from build123d import *

# Parameters (mm, degrees)
SKETCH1_R           = 17
BOSS_EXTRUDE1_DEPTH = 15
CUT_EXTRUDE2_DEPTH  = 5
SKETCH3_R           = 1.75
CUT_EXTRUDE3_DEPTH  = 5
SKETCH4_W           = 3
SKETCH4_H           = 4
SKETCH5_R           = 6.36
CUT_EXTRUDE4_DEPTH  = 3.3


with BuildPart() as part:
    # Sketch1 → Boss-Extrude1 (new body)
    with BuildSketch(Plane.XY):
        Circle(SKETCH1_R)
    extrude(amount=BOSS_EXTRUDE1_DEPTH)

    # Sketch2 → Cut-Extrude2 (cut)
    with BuildSketch(Plane(origin=(0, 0, 0), x_dir=(-1, 0, 0), z_dir=(0, 0, -1))):
        with BuildLine():
            ThreePointArc((5.676819497, 7.303165094), (3.539821749, 8.545885676), (1.15, 9.178235124))
            ThreePointArc((1.15, 9.178235124), (0, 8.028235124), (-1.15, 9.178235124))
            ThreePointArc((-1.15, 9.178235124), (-3.539821749, 8.545885676), (-5.676819497, 7.303165094))
            ThreePointArc((-5.676819497, 7.303165094), (-5.676819497, 5.676819497), (-7.303165094, 5.676819497))
            ThreePointArc((-7.303165094, 5.676819497), (-8.545885676, 3.539821749), (-9.178235124, 1.15))
            ThreePointArc((-9.178235124, 1.15), (-8.028235124, 0), (-9.178235124, -1.15))
            ThreePointArc((-9.178235124, -1.15), (-8.545885676, -3.539821749), (-7.303165094, -5.676819497))
            ThreePointArc((-7.303165094, -5.676819497), (-5.676819497, -5.676819497), (-5.676819497, -7.303165094))
            ThreePointArc((-5.676819497, -7.303165094), (-3.539821749, -8.545885676), (-1.15, -9.178235124))
            ThreePointArc((-1.15, -9.178235124), (0, -8.028235124), (1.15, -9.178235124))
            ThreePointArc((1.15, -9.178235124), (3.539821749, -8.545885676), (5.676819497, -7.303165094))
            ThreePointArc((5.676819497, -7.303165094), (5.676819497, -5.676819497), (7.303165094, -5.676819497))
            ThreePointArc((7.303165094, -5.676819497), (8.545885676, -3.539821749), (9.178235124, -1.15))
            ThreePointArc((9.178235124, -1.15), (8.028235124, 0), (9.178235124, 1.15))
            ThreePointArc((9.178235124, 1.15), (8.545885676, 3.539821749), (7.303165094, 5.676819497))
            ThreePointArc((7.303165094, 5.676819497), (5.676819497, 5.676819497), (5.676819497, 7.303165094))
        make_face()
        with BuildLine():
            Line((9.333809512, 10.960155108), (5.676819497, 7.303165094))
            ThreePointArc((5.676819497, 7.303165094), (6.540737726, 6.540737726), (7.303165094, 5.676819497))
            Line((7.303165094, 5.676819497), (10.960155108, 9.333809512))
            ThreePointArc((10.960155108, 9.333809512), (10.960155108, 10.960155108), (9.333809512, 10.960155108))
        make_face()
        with BuildLine():
            Line((14.35, 1.15), (9.178235124, 1.15))
            ThreePointArc((9.178235124, 1.15), (9.232041348, 0.57611852), (9.25, 0))
            ThreePointArc((9.25, 0), (9.232041348, -0.57611852), (9.178235124, -1.15))
            Line((9.178235124, -1.15), (14.35, -1.15))
            ThreePointArc((14.35, -1.15), (15.5, 0), (14.35, 1.15))
        make_face()
        with BuildLine():
            Line((10.960155108, -9.333809512), (7.303165094, -5.676819497))
            ThreePointArc((7.303165094, -5.676819497), (6.540737726, -6.540737726), (5.676819497, -7.303165094))
            Line((5.676819497, -7.303165094), (9.333809512, -10.960155108))
            ThreePointArc((9.333809512, -10.960155108), (10.960155108, -10.960155108), (10.960155108, -9.333809512))
        make_face()
        with BuildLine():
            Line((1.15, -14.35), (1.15, -9.178235124))
            ThreePointArc((1.15, -9.178235124), (0, -9.25), (-1.15, -9.178235124))
            Line((-1.15, -9.178235124), (-1.15, -14.35))
            ThreePointArc((-1.15, -14.35), (0, -15.5), (1.15, -14.35))
        make_face()
        with BuildLine():
            ThreePointArc((-5.676819497, -7.303165094), (-6.540737726, -6.540737726), (-7.303165094, -5.676819497))
            Line((-7.303165094, -5.676819497), (-10.960155108, -9.333809512))
            ThreePointArc((-10.960155108, -9.333809512), (-10.960155108, -10.960155108), (-9.333809512, -10.960155108))
            Line((-9.333809512, -10.960155108), (-5.676819497, -7.303165094))
        make_face()
        with BuildLine():
            ThreePointArc((-9.178235124, -1.15), (-9.25, 0), (-9.178235124, 1.15))
            Line((-9.178235124, 1.15), (-14.35, 1.15))
            ThreePointArc((-14.35, 1.15), (-15.5, 0), (-14.35, -1.15))
            Line((-14.35, -1.15), (-9.178235124, -1.15))
        make_face()
        with BuildLine():
            ThreePointArc((-7.303165094, 5.676819497), (-6.540737726, 6.540737726), (-5.676819497, 7.303165094))
            Line((-5.676819497, 7.303165094), (-9.333809512, 10.960155108))
            ThreePointArc((-9.333809512, 10.960155108), (-10.960155108, 10.960155108), (-10.960155108, 9.333809512))
            Line((-10.960155108, 9.333809512), (-7.303165094, 5.676819497))
        make_face()
        with BuildLine():
            Line((1.15, 9.178235124), (1.15, 14.35))
            ThreePointArc((1.15, 14.35), (0, 15.5), (-1.15, 14.35))
            Line((-1.15, 14.35), (-1.15, 9.178235124))
            ThreePointArc((-1.15, 9.178235124), (0, 9.25), (1.15, 9.178235124))
        make_face()
        with BuildLine():
            ThreePointArc((5.676819497, -7.303165094), (6.540737726, -6.540737726), (7.303165094, -5.676819497))
            ThreePointArc((7.303165094, -5.676819497), (5.676819497, -5.676819497), (5.676819497, -7.303165094))
        make_face()
        with BuildLine():
            ThreePointArc((-1.15, 9.178235124), (0, 8.028235124), (1.15, 9.178235124))
            ThreePointArc((1.15, 9.178235124), (0, 9.25), (-1.15, 9.178235124))
        make_face()
        with BuildLine():
            ThreePointArc((7.303165094, 5.676819497), (6.540737726, 6.540737726), (5.676819497, 7.303165094))
            ThreePointArc((5.676819497, 7.303165094), (5.676819497, 5.676819497), (7.303165094, 5.676819497))
        make_face()
        with BuildLine():
            ThreePointArc((9.25, 0), (9.232041348, 0.57611852), (9.178235124, 1.15))
            ThreePointArc((9.178235124, 1.15), (8.028235124, 0), (9.178235124, -1.15))
            ThreePointArc((9.178235124, -1.15), (9.232041348, -0.57611852), (9.25, 0))
        make_face()
        with BuildLine():
            ThreePointArc((-1.15, -9.178235124), (0, -9.25), (1.15, -9.178235124))
            ThreePointArc((1.15, -9.178235124), (0, -8.028235124), (-1.15, -9.178235124))
        make_face()
        with BuildLine():
            ThreePointArc((-5.676819497, -7.303165094), (-5.676819497, -5.676819497), (-7.303165094, -5.676819497))
            ThreePointArc((-7.303165094, -5.676819497), (-6.540737726, -6.540737726), (-5.676819497, -7.303165094))
        make_face()
        with BuildLine():
            ThreePointArc((-9.178235124, -1.15), (-8.028235124, 0), (-9.178235124, 1.15))
            ThreePointArc((-9.178235124, 1.15), (-9.25, 0), (-9.178235124, -1.15))
        make_face()
        with BuildLine():
            ThreePointArc((-7.303165094, 5.676819497), (-5.676819497, 5.676819497), (-5.676819497, 7.303165094))
            ThreePointArc((-5.676819497, 7.303165094), (-6.540737726, 6.540737726), (-7.303165094, 5.676819497))
        make_face()
    extrude(amount=-CUT_EXTRUDE2_DEPTH, mode=Mode.SUBTRACT)

    # Sketch3 → Cut-Extrude3 (cut)
    with BuildSketch(Plane.XY.offset(15)):
        with Locations((0, 9.78)):
            Circle(SKETCH3_R)
        with Locations((9.78, 0)):
            Circle(SKETCH3_R)
        with Locations((0, -9.78)):
            Circle(SKETCH3_R)
        with Locations((-9.78, 0)):
            Circle(SKETCH3_R)
    extrude(amount=-CUT_EXTRUDE3_DEPTH, mode=Mode.SUBTRACT)

    # Sketch4 → Revolve1 (revolve)
    with BuildSketch(Plane(origin=(0, 0, 0), x_dir=(0, 0, -1), z_dir=(1, 0, 0))):
        with Locations((-7.5, -19)):
            Rectangle(SKETCH4_W, SKETCH4_H)
    revolve(axis=Axis((0, 0, 20.375620023), (0, 0, -1)))

    # Sketch5 → Cut-Extrude4 (cut)
    with BuildSketch(Plane.XY.offset(15)):
        Circle(SKETCH5_R)
    extrude(amount=-CUT_EXTRUDE4_DEPTH, mode=Mode.SUBTRACT)


solid = part.part
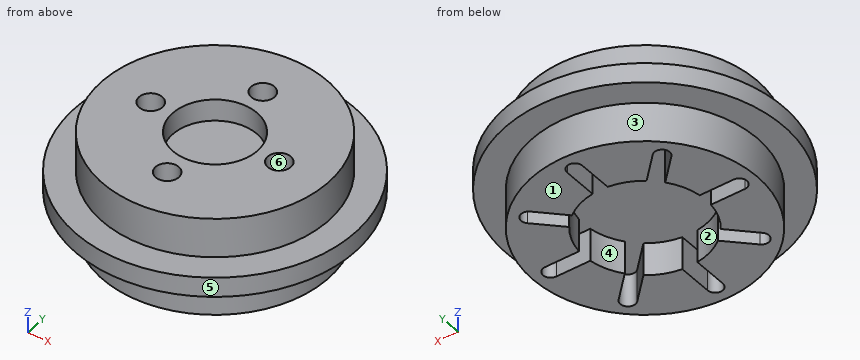
The model under review builds one solid part; all positions refer to its coordinate system, in mm. Face numbers are marked on the shaded views. A direction names the side the tool comes from. Coordinates: 2 decimals unless noted, no trailing zeros. Loops run counter-clockwise (first coordinate to the right, second up) from the corner with the lowest first, then second, coordinate; pieces in that order, holes last. Notation, with made-up numbers: (-29.75, 52) -> (23.25, 52) arc R16 cw to (23.25, 57) -> close; hole circle Ø9 at (-26.75, 9). An arc over 180 degrees is marked (long way). Use a Markdown table: item, result. Add a question column.
1. Add section D-D on y = 4. Write out the cut boundary in (x, z).
2. Add section C-C on z = 12.5. Write out the cut boundary in (x, y).
3. To check wall thickness, follow line 1 (Y direction, x = 0, z = 11.75); line 2 (X direction, y = -11, z = 4); line 3 (Y direction, x = 8, z = 1.5). State the ranges of each line that lie inside material, in increasing order.
4. Clearance check with flat-ended pins moving along their axes: pin 1 Ø1 at (x, z) = (-15.5, 12) entering from -Y; pin 2 Ø10 at (x, y) = (0, 0) entering from -Z; pin 3 Ø3 at (x, y) = (-9.78, 0) entering from +Z. State where each tip first meets the part, or that it passes through.
5. Machinability: for the marked faces 4, 5 and 6, which of the approach directions +Z, -Z, +X, -X, +Y, -Y give a long, thin tool a straight path to every point of the face, cutting with its end or side? Answer none if there is none.
6. Add section A-A on x = 0. Write out the cut boundary in (y, z), plus the area to 3 significant figures.
7. Draft analysis for pull direction X (two halves, no side actions). For the marked faces 1, 2 and 3, state which applies: pulls with the +X half, pulls with the -X half, needs draft (parallel to the pull), parting line crosses it, or undercut.
Returned:
| question | item | result |
|---|---|---|
| 1 | outline | (-20.62, 6) -> (-16.52, 6) -> (-16.52, 0) -> (-8.34, 0) -> (-8.34, 5) -> (8.34, 5) -> (8.34, 0) -> (16.52, 0) -> (16.52, 6) -> (20.62, 6) -> (20.62, 9) -> (16.52, 9) -> (16.52, 15) -> (4.94, 15) -> (4.94, 11.7) -> (-4.94, 11.7) -> (-4.94, 15) -> (-16.52, 15) -> (-16.52, 9) -> (-20.62, 9) -> close |
| 2 | outline | circle Ø34 at (0, 0); hole circle Ø3.5 at (-9.78, 0); hole circle Ø12.72 at (0, 0); hole circle Ø3.5 at (0, -9.78); hole circle Ø3.5 at (0, 9.78); hole circle Ø3.5 at (9.78, 0) |
| 3 | line 1 | y = -17 to -11.53, -8.03 to -6.36, 6.36 to 8.03, 11.53 to 17 |
| 3 | line 2 | x = -12.96 to -10.92, -9.38 to -1.15, 1.15 to 9.38, 10.92 to 12.96 |
| 3 | line 3 | y = -15 to -9.63, -6.37 to -4.64, 4.64 to 6.37, 9.63 to 15 |
| 4 | pin 1 | stops at y = -8 |
| 4 | pin 2 | stops at z = 5 |
| 4 | pin 3 | stops at z = 10 |
| 5 | face 4 | -Z |
| 5 | face 5 | +Z, -Z |
| 5 | face 6 | +Z |
| 6 | outline | (-21, 6) -> (-17, 6) -> (-17, 0) -> (-15.5, 0) -> (-15.5, 5) -> (15.5, 5) -> (15.5, 0) -> (17, 0) -> (17, 6) -> (21, 6) -> (21, 9) -> (17, 9) -> (17, 15) -> (11.53, 15) -> (11.53, 10) -> (8.03, 10) -> (8.03, 15) -> (6.36, 15) -> (6.36, 11.7) -> (-6.36, 11.7) -> (-6.36, 15) -> (-8.03, 15) -> (-8.03, 10) -> (-11.53, 10) -> (-11.53, 15) -> (-17, 15) -> (-17, 9) -> (-21, 9) -> close |
| 6 | area | 302 mm² |
| 7 | face 1 | needs draft |
| 7 | face 2 | undercut |
| 7 | face 3 | parting line crosses it |
